The listing builds one solid part. Answer for the finished solid, in the listing's coordinates (mm). Face numbers are marked on the shaded views. A direction names the side the tool comes from. Give positions to 0.01 mm unless a question says otherwise; leave off trailing zeros. Loops run counter-clockwise (first coordinate to the right, second up) from the corner with the lowest first, then second, coordinate; pieces in that order, holes last. Notation, with made-up numbers: (-9, 52.5) -> (50, 52.5) arc R27 ccw to (50, 87.5) -> close; hole circle Ø1 at (-8.75, 78.25). An arc over 180 degrees is marked (long way). One line per question, with ' | ' between items. Start each with the question number.
from build123d import *

# Parameters (mm, degrees)
BASEHEAD_DEPTH = 4.7752


with BuildPart() as part:
    # Sketch1 → BaseHead (new body)
    with BuildSketch(Plane(origin=(0, 0, 0), x_dir=(0, 0, -1), z_dir=(1, 0, 0))):
        Polygon((5.5626, 3.211568607), (5.5626, -3.211568607), (0, -6.423137215), (-5.5626, -3.211568607), (-5.5626, 3.211568607), (0, 6.423137215), align=None)
    extrude(amount=BASEHEAD_DEPTH)

    # BodySke → BaseBody (revolve)
    with BuildSketch(Plane.XY):
        Polygon((0, 0), (30.1752, 0), (30.1752, 2.41935), (29.41955, 3.175), (0, 3.175), align=None)
    revolve(axis=Axis((0, 0, 0), (1, 0, 0)))

    # Sketch3 → HeadChamfer (revolve, cut)
    with BuildSketch(Plane.XY):
        Polygon((0, 5.5626), (4.163005602, 12.773137215), (4.163005602, 19.123137215), (-12.7, 19.123137215), (-12.7, 5.5626), align=None)
    revolve(axis=Axis((0, 0, 0), (1, 0, 0)), mode=Mode.SUBTRACT)


solid = part.part
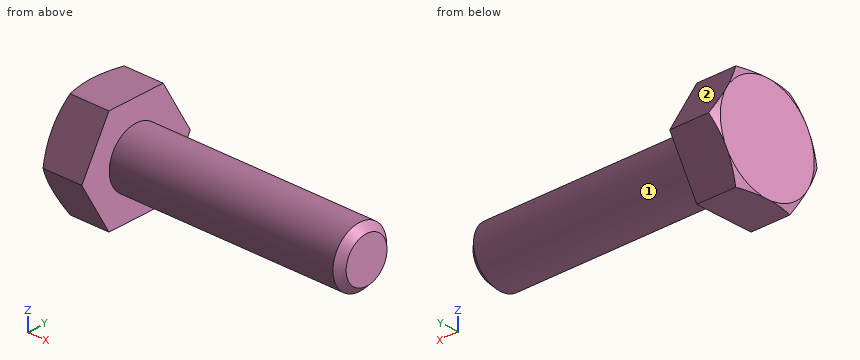
1. Straight lines are drawn through the part: L1, parallel to X at y = -1.5, z = -4.25; L2, parallel to Z at x = 5.5, y = -0.25; L3, parallel to Z at x = 16, y = 1.75. For each, find the intervals that lie inside material, in ascending order.
2. For the marked faces 1 and 2, determine the directions among +Z, -Z, +X, -X, +Y, -Y from which every point of the face is accessible in a straight line to the end or side of a thin tool.
3. Each of these flat-tipped pins is pushed along its axis until it touches: pin 1 Ø1.5 at (x, z) = (12, 3) entering from +Y; pin 2 Ø3 at (x, y) = (25.5, 4) entering from +Z; pin 3 Ø1 at (x, y) = (25.5, 0.5) entering from +Z (3 decimals). Where does it stop, or does it pass through?
4. The part is cut by section A-A (x = 18). Write down the section's boundary in (y, z) (3 decimals), plus the area to 3 significant figures.
Check sheet entries:
1) L1: x = 0 to 4.78 | L2: z = -3.17 to 3.17 | L3: z = -2.65 to 2.65
2) face 1: +X | face 2: +Z, +X, -X, +Y
3) pin 1: stops at y = 2.24 | pin 2: stops at z = 1.96 | pin 3: stops at z = 3.175
4) outline: circle Ø6.35 at (0, 0) | area: 31.7 mm^2
